from build123d import *

# Parameters (mm, degrees)
F3_D     = 5
F3_DEPTH = 9
F3_TIP   = 1.5021515476
F4_D     = 6
F4_DEPTH = 6.2
F4_TIP   = 1.8025818571


with BuildPart() as f1:
    # F0 (on Front) → F1 (revolve)
    with BuildSketch(Plane.XZ):
        Polygon((0, 24), (0, 0), (45, 0), (45, 15.2679491924), (44, 17), (44, 20), (42.2679491924, 20), (39.9585481157, 24), (31.5, 24), (31.5, 30.1464466094), (31.1464466094, 30.5), (16.1035533906, 30.5), (15.75, 30.1464466094), (15.75, 24), align=None)
    revolve(axis=Axis((0, 0, 12), (0, 0, -1)))

    # F3
    with Locations(Plane.XY.offset(30.5)):
        with Locations((-17.6776695297, 17.6776695297), (-17.6776695297, -17.6776695297), (17.6776695297, 17.6776695297), (17.6776695297, -17.6776695297)):
            Hole(F3_D / 2, depth=F3_DEPTH)
            with Locations((0, 0, -(F3_DEPTH + F3_TIP / 2))):  # 118° drill point
                Cone(0, F3_D / 2, F3_TIP, mode=Mode.SUBTRACT)

    # F4
    with Locations(Plane.XY.offset(30.5)):
        with Locations((-25, 0)):
            Hole(F4_D / 2, depth=F4_DEPTH)
            with Locations((0, 0, -(F4_DEPTH + F4_TIP / 2))):  # 118° drill point
                Cone(0, F4_D / 2, F4_TIP, mode=Mode.SUBTRACT)


solid = f1.part
Build history of the part. All positions in model axes, mm. A direction names the side the tool comes from. Round coordinates to 2 decimals unless told otherwise and drop trailing zeros. Write each loop counter-clockwise with the first axis right and the second up, starting at its lowest first coordinate (ties: lowest second). Pieces come first, ordered by that corner, then holes. Notation, with made-up numbers: M -13,38 L 16,38 A32 ccw 16,64 Z; hole C 32,8.25 d7. An arc over 180 degrees is marked long. Answer in a Markdown table with one row per item.
1. Saw through at A-A (z = 11). List the corners of the cut face in (x, y).
Geometry check:
| item | result |
|---|---|
| outline | C 0,0 d90 |
2. Flat gauge pins, fed straight in: P1, Ø4.5, axis at x = 17.68, y = 17.68, coming from the -Z side; P2, Ø6, axis at y = -20, z = 8, coming from the +X side; P3, Ø1.5, axis at x = 27.5, z = 7.5, coming from the -Y side; P4, Ø6, axis at x = 5.5, z = 12, coming from the -Y side. Where does each tip first touch, or does it go through?
Geometry check:
| item | result |
|---|---|
| P1 | z = 0 |
| P2 | x = 41.67 |
| P3 | y = -36.19 |
| P4 | y = -44.93 |
3. Probe L1, parallel to X at y = 0, z = 26.5; L2, parallel to Y at x = -16, z = 23; L3, parallel to Y at x = 0, z = 26.5. List the from-to ranges inside material, lowest first. Write a range as [from, to].
Geometry check:
| item | result |
|---|---|
| L1 | [-31.5, -28], [-22, -15.75], [15.75, 31.5] |
| L2 | [-37.24, -19.53], [-15.82, 15.82], [19.53, 37.24] |
| L3 | [-31.5, -15.75], [15.75, 31.5] |
4. Mould opens along X. For faces 1 (the face through (18.08, -17.84, 20.26)), 2 (the face through (-4.101, -31.232, 27.116)), 3 (the face through (1, -1, 0)), 4 (the face through (-22, 0, 27)) say: +X half, -X half, draft (parallel to the pull), parting line (faces both ways), or undercut.
Geometry check:
| item | result |
|---|---|
| face 1 | undercut |
| face 2 | parting line |
| face 3 | draft |
| face 4 | undercut |
5. Which spindle directions (+Z, -Z, +X, -X, +Y, -Y) get a long thin tool onto all of the face, cutting with end or side? Do faces 5 (the face through (13, 13, 30.5)), 6 (the face through (19.52, -15.99, 25.94)). Say none if no direction does.
Geometry check:
| item | result |
|---|---|
| face 5 | +Z, +X, -X, +Y, -Y |
| face 6 | +Z |
